Geometry: final body of the model. Coordinates: model frame, mm. Give positions to 0.01 mm unless a question says otherwise; leave off trailing zeros. Order: outer loops, then holes, each group sorted by start corner. A loop starts at its lowest first (then second) coordinate and runs counter-clockwise, first axis right, second up. Notation, with made-up numbers: (-5, 18.25) -> (40, 18.25) arc R21 ccw to (40, 22.25) -> close; hole circle Ø8 at (78, 57.5). An arc over 180 degrees is marked (long way). One line per question, with ' | ' between items. Start each with the question number.
(1) Section A-A (y = 197). Return loops of the section in (x, z).
(2) Section D-D (z = 1.2). State how many separate pieces and enclosed holes the cut face has, then the cut area to 3 significant figures.
(3) Section C-C (x = 355.5). Return loops of the section in (y, z).
(4) Section B-B (x = 343). Return loops of the section in (y, z), then the cut area to 3 significant figures.
(5) First-contact query: pin 1 Ø10 at (x, y) = (317, 201.5) entering from -Z; pin 2 Ø1.8 at (x, z) = (327, 4) entering from +Y; pin 3 Ø4 at (x, y) = (273.71, 172.11) entering from -Z; pin 4 Ø1.5 at (x, z) = (360, 4) entering from +Y. Flat tips, straight axial feed; report the tip coordinate or a pass-through.
(6) Ray query, L1, parallel to X at y = 217, z = 3.8; L2, parallel to X at y = 195.5, z = 3.15; L3, parallel to X at y = 189, z = 3.3. Return the intervals inside material, ascending.
```python
from build123d import *

# Parameters (mm, degrees)
SKETCH1_R           = 2.281562065
SKETCH1_R_2         = 2.125
SKETCH1_W           = 5.9944
SKETCH1_H           = 12.7
SKETCH1_W_2         = 5.986441201
SKETCH1_H_2         = 12.703753504
SKETCH1_W_3         = 5.986441202
BOSS_EXTRUDE1_DEPTH = 5.9944


with BuildPart() as part:
    # Sketch1 → Boss-Extrude1 (new body)
    with BuildSketch(Plane.XY):
        with BuildLine():
            Line((270.254984812, 144.069366267), (333.659384812, 144.069366267))
            Line((333.659384812, 144.069366267), (339.653784812, 144.069366267))
            Line((339.653784812, 144.069366267), (375.974984812, 144.069366267))
            ThreePointArc((375.974984812, 144.069366267), (377.771036036, 144.813315043), (378.514984812, 146.609366267))
            Line((378.514984812, 146.609366267), (378.514984812, 226.632730682))
            ThreePointArc((378.514984812, 226.632730682), (377.770473259, 228.429344507), (375.973393287, 229.172730183))
            Line((375.973393287, 229.172730183), (347.813544609, 229.155085658))
            Line((347.813544609, 229.155085658), (347.813544609, 216.451324674))
            Line((347.813544609, 216.451324674), (341.815166975, 216.451324674))
            Line((341.815166975, 216.451324674), (341.815166975, 229.155085658))
            Line((341.815166975, 229.155085658), (330.740769149, 229.140627138))
            Line((330.740769149, 229.140627138), (330.740769149, 216.444385628))
            Line((330.740769149, 216.444385628), (324.738412704, 216.444385628))
            Line((324.738412704, 216.444385628), (324.738412704, 229.140627138))
            Line((324.738412704, 229.140627138), (318.219144609, 229.136542265))
            Line((318.219144609, 229.136542265), (318.219144609, 216.431429486))
            Line((318.219144609, 216.431429486), (312.224744609, 216.431429486))
            Line((312.224744609, 216.431429486), (312.224744609, 229.131429486))
            Line((312.224744609, 229.131429486), (270.25739927, 229.171322574))
            ThreePointArc((270.25739927, 229.171322574), (268.45978743, 228.428228383), (267.714984812, 226.631323721))
            Line((267.714984812, 226.631323721), (267.714984812, 146.609366267))
            ThreePointArc((267.714984812, 146.609366267), (268.458933587, 144.813315043), (270.254984812, 144.069366267))
        make_face()
        with Locations((273.714984812, 148.112259486)):
            Circle(SKETCH1_R, mode=Mode.SUBTRACT)
        with Locations((291.714984812, 148.112259486)):
            Circle(SKETCH1_R_2, mode=Mode.SUBTRACT)
        with Locations((273.714984812, 172.112259486)):
            Circle(SKETCH1_R_2, mode=Mode.SUBTRACT)
        with Locations((291.714984812, 172.112259486)):
            Circle(SKETCH1_R_2, mode=Mode.SUBTRACT)
        Polygon((273.709384812, 179.000344994), (273.709384812, 186.620344994), (273.709384812, 194.240344994), (280.059384812, 194.240344994), (280.059384812, 179.000344994), align=None, mode=Mode.SUBTRACT)
        with Locations((315.221944609, 169.781429486)):
            Rectangle(SKETCH1_W, SKETCH1_H, mode=Mode.SUBTRACT)
        with Locations((354.514984812, 148.112259486)):
            Circle(SKETCH1_R_2, mode=Mode.SUBTRACT)
        with Locations((372.514984812, 148.112259486)):
            Circle(SKETCH1_R_2, mode=Mode.SUBTRACT)
        with Locations((327.771421413, 171.992516355)):
            Rectangle(SKETCH1_W_2, SKETCH1_H_2, mode=Mode.SUBTRACT)
        with Locations((344.840218063, 172.003211399)):
            Rectangle(SKETCH1_W_3, SKETCH1_H_2, mode=Mode.SUBTRACT)
        with Locations((354.514984812, 172.112259486)):
            Circle(SKETCH1_R_2, mode=Mode.SUBTRACT)
        with Locations((372.514984812, 172.112259486)):
            Circle(SKETCH1_R_2, mode=Mode.SUBTRACT)
        Polygon((372.520584812, 186.620344994), (372.520584812, 179.000344994), (366.170584812, 179.000344994), (366.170584812, 194.240344994), (372.520584812, 194.240344994), align=None, mode=Mode.SUBTRACT)
        with Locations((273.714984812, 201.131429486)):
            Circle(SKETCH1_R_2, mode=Mode.SUBTRACT)
        with Locations((291.714984812, 201.131429486)):
            Circle(SKETCH1_R_2, mode=Mode.SUBTRACT)
        with Locations((315.221944609, 196.281429486)):
            Rectangle(SKETCH1_W, SKETCH1_H, mode=Mode.SUBTRACT)
        with Locations((273.714984812, 225.131429486)):
            Circle(SKETCH1_R_2, mode=Mode.SUBTRACT)
        with Locations((291.714984812, 225.131429486)):
            Circle(SKETCH1_R_2, mode=Mode.SUBTRACT)
        with Locations((327.75550617, 197.392511369)):
            Rectangle(SKETCH1_W_3, SKETCH1_H_2, mode=Mode.SUBTRACT)
        with Locations((344.82430282, 197.403206413)):
            Rectangle(SKETCH1_W_2, SKETCH1_H_2, mode=Mode.SUBTRACT)
        with Locations((354.514984812, 201.131429486)):
            Circle(SKETCH1_R_2, mode=Mode.SUBTRACT)
        with Locations((372.514984812, 201.131429486)):
            Circle(SKETCH1_R_2, mode=Mode.SUBTRACT)
        with Locations((354.514984812, 225.131429486)):
            Circle(SKETCH1_R_2, mode=Mode.SUBTRACT)
        with Locations((372.514984812, 225.131429486)):
            Circle(SKETCH1_R_2, mode=Mode.SUBTRACT)
    extrude(amount=BOSS_EXTRUDE1_DEPTH)


solid = part.part
```
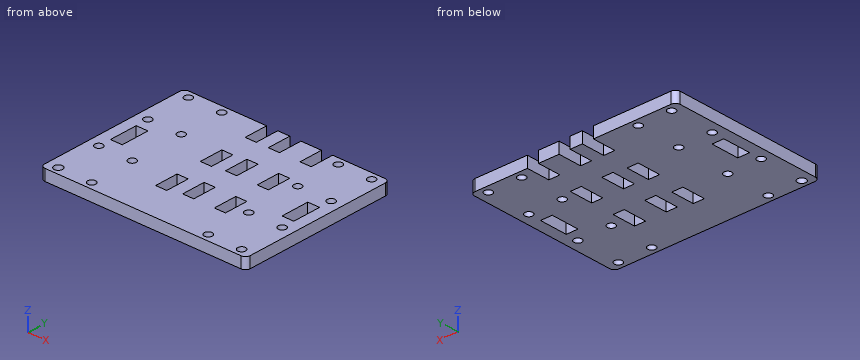
Response:
1) outline: (267.71, 0) -> (312.22, 0) -> (312.22, 5.99) -> (267.71, 5.99) -> close; (318.22, 0) -> (324.76, 0) -> (324.76, 5.99) -> (318.22, 5.99) -> close; (330.75, 0) -> (341.83, 0) -> (341.83, 5.99) -> (330.75, 5.99) -> close; (347.82, 0) -> (378.51, 0) -> (378.51, 5.99) -> (347.82, 5.99) -> close
2) separate pieces: 1 | enclosed holes: 24 | area: 8,310 mm^2
3) outline: (144.07, 0) -> (146.23, 0) -> (146.23, 5.99) -> (144.07, 5.99) -> close; (150, 0) -> (170.23, 0) -> (170.23, 5.99) -> (150, 5.99) -> close; (174, 0) -> (199.25, 0) -> (199.25, 5.99) -> (174, 5.99) -> close; (203.01, 0) -> (223.25, 0) -> (223.25, 5.99) -> (203.01, 5.99) -> close; (227.01, 0) -> (229.16, 0) -> (229.16, 5.99) -> (227.01, 5.99) -> close
4) outline: (144.07, 0) -> (165.65, 0) -> (165.65, 5.99) -> (144.07, 5.99) -> close; (178.36, 0) -> (191.05, 0) -> (191.05, 5.99) -> (178.36, 5.99) -> close; (203.76, 0) -> (216.45, 0) -> (216.45, 5.99) -> (203.76, 5.99) -> close | area: 282 mm^2
5) pin 1: stops at z = 0 | pin 2: stops at y = 216.44 | pin 3: passes through | pin 4: stops at y = 229.16
6) L1: x = 267.71 to 312.22, 318.22 to 324.74, 330.74 to 341.82, 347.81 to 378.51 | L2: x = 267.71 to 312.22, 318.22 to 324.76, 330.75 to 341.83, 347.82 to 378.51 | L3: x = 267.71 to 273.71, 280.06 to 366.17, 372.52 to 378.51
